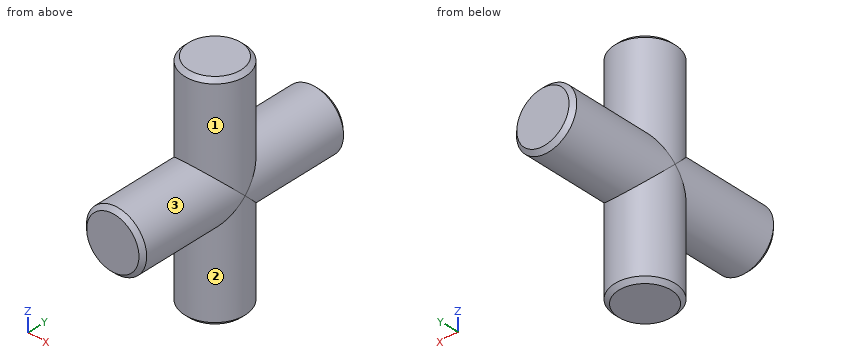
```python
from build123d import *

# Parameters (mm, degrees)
SKETCH_1_R      = 1.5
EXTRUDE_1_DEPTH = 11
SKETCH_2_R      = 1.5
EXTRUDE_2_DEPTH = 5.5
CHAMFER_1_SIZE  = 0.2


with BuildPart() as part:
    # 草图1 → 凸台-拉伸1 (new body)
    with BuildSketch(Plane(origin=(0, 0, 0), x_dir=(1, 0, 0), z_dir=(0, 1, 0))):
        Circle(SKETCH_1_R)
    extrude(amount=EXTRUDE_1_DEPTH)

    # 草图2 → 凸台-拉伸2 (add, symmetric)
    with BuildSketch(Plane.XY):
        with Locations((0, 5.5)):
            Circle(SKETCH_2_R)
    extrude(amount=EXTRUDE_2_DEPTH, both=True)

    # 倒角1
    chamfer_1_edges = [part.edges().sort_by_distance(p)[0] for p in [
        (-1.5, 0, 0),
        (-1.5, 11, 0),
        (-1.5, 5.5, -5.5),
        (-1.5, 5.5, 5.5),
    ]]
    chamfer(chamfer_1_edges, length=CHAMFER_1_SIZE)


solid = part.part
```
Can you work these out from the model? Positions are in its coordinate system, mm. Face numbers are marked on the shaded views. A direction names the side the tool comes from. Coordinates: 2 decimals unless noted, no trailing zeros. Order: outer loops, then holes, each group sorted by start corner. A loop starts at its lowest first (then second) coordinate and runs counter-clockwise, first axis right, second up.
1. If we section it at C-C (y = 1): Please give me the cut outline in (x, z), then the cut area to 3 significant figures.
2. I need wall thicknesses on line 1 (Z direction, x = -1.1, y = 3.25); line 2 (Y direction, x = 0.05, z = -3.25); line 3 (X direction, y = 9.25, z = 0.25). Which ranges of each line are inside material? Lowest first, please.
3. For the marked faces 1, 2 and 3, which set-ups out of +Z, -Z, +X, -X, +Y, -Y let a thin tool reach every point of the face, with its end or its side?
4. If we section it at B-B (z = -3.75): Please give me the cut outline in (x, y).
5. I'm going to push a flat-ended pin straight in: pin 1 (1 mm diameter, centred on y = 1.5, z = -3.5, fed in from -X). Where does the tip first touch, or does it pass through?
6. If we section it at A-A (x = 0): Please give me the cut outline in (y, z).
Entries:
1. outline: circle Ø3 at (0, 0)
1. area: 7.07 mm2
2. line 1: z = -1.02 to 1.02
2. line 2: y = 4 to 7
2. line 3: x = -1.48 to 1.48
3. face 1: +Z
3. face 2: -Z
3. face 3: -Y
4. outline: circle Ø3 at (0, 5.5)
5. pin 1: passes through
6. outline: (0, -1.3) - (0.2, -1.5) - (4, -1.5) - (4, -5.3) - (4.2, -5.5) - (6.8, -5.5) - (7, -5.3) - (7, -1.5) - (10.8, -1.5) - (11, -1.3) - (11, 1.3) - (10.8, 1.5) - (7, 1.5) - (7, 5.3) - (6.8, 5.5) - (4.2, 5.5) - (4, 5.3) - (4, 1.5) - (0.2, 1.5) - (0, 1.3) - close
